Read the model definition and answer for the solid it produces. Units are mm, in the model's axes. Round coordinates to 2 decimals unless told otherwise and drop trailing zeros. Order: outer loops, then holes, each group sorted by start corner. A loop starts at its lowest first (then second) coordinate and runs counter-clockwise, first axis right, second up. Notation, with made-up numbers: (10.25, 70) -> (68.25, 70) arc R9 cw to (68.25, 75) -> close; hole circle Ø2 at (-1, 53). An arc over 180 degrees is marked (long way). Use a Markdown table: item, result. Add a question column.
1. Section C-C, the plane x = -8.5 is taken. Give the vertices of the cut face in (y, z).
2. Section D-D, the plane x = 59.5 is taken. Give the vertices of the cut face in (y, z).
3. Consider L1, parallel to Y at x = -7.5, z = 3.95; L2, parallel to Y at x = 8, z = 3.8; L3, parallel to Y at x = -13.5, z = 3.3. Determine where each line is inside the solid, lowest interval first. Write a range as [from, to].
4. Section A-A, the plane x = 12.5 is taken. Give the vertices of the cut face in (y, z).
5. Given pin 1 (2.5 mm diameter, centred on y = -155, z = 2, fed in from +X); pin 2 (2.5 mm diameter, centred on x = -36, z = 2.5, fed in from -Y); pin 3 (2 mm diameter, centred on x = -61.5, z = 3, fed in from -Y); pin 4 (2.5 mm diameter, centred on x = -63.46, y = -187.43, fed in from +Z), each flat-ended and moving along its own axis, determine where each tip first touches the part or whether it passes through.
6. Section B-B, the plane z = 2.8 is taken. Give the number of separate pieces and of enclosed holes in the cut face, then the cut area to 3 significant figures.
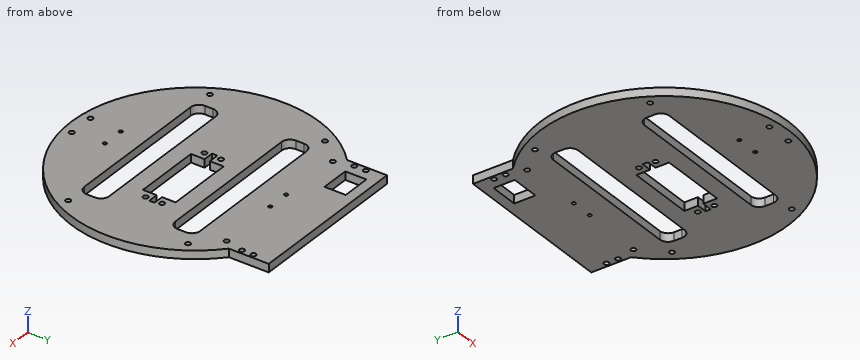
```python
from build123d import *

# Parameters (mm, degrees)
RESSALTO_EXTRUS_O1_DEPTH = 5
ESBO_O2_R                = 1.5
CORTE_EXTRUS_O1_DEPTH    = 10
ESBO_O3_W                = 6.3
ESBO_O3_H                = 3.2
ESBO_O3_R                = 1.5
CORTE_EXTRUS_O2_DEPTH    = 10
ESBO_O4_W                = 17.5
ESBO_O4_H                = 12.8
CORTE_EXTRUS_O3_DEPTH    = 6
ESBO_O5_R                = 1.5
CORTE_EXTRUS_O4_DEPTH    = 10
ESBO_O6_R                = 1.05
CORTE_EXTRUS_O5_DEPTH    = 10
CORTE_EXTRUS_O6_DEPTH    = 6


with BuildPart() as part:
    # Esboço1 → Ressalto-extrusão1 (new body)
    with BuildSketch(Plane.XY):
        with BuildLine():
            Line((44.495405461, -168.430491325), (44.495405461, -144.332190763))
            Line((44.495405461, -144.332190763), (-55.573351401, -144.332190763))
            Line((-55.573351401, -144.332190763), (-55.573351401, -168.393072388))
            Line((-55.573351401, -168.393072388), (-55.504594539, -168.430491325))
            ThreePointArc((-55.504594539, -168.430491325), (-5.504594539, -299.332190763), (44.495405461, -168.430491325))
        make_face()
    extrude(amount=RESSALTO_EXTRUS_O1_DEPTH)

    # Esboço2 → Corte-extrusão1 (cut)
    with BuildSketch(Plane.XY.offset(5)):
        with Locations((39.44625518, -173.430491325)):
            Circle(ESBO_O2_R)
        with Locations((52.44625518, -187.430491325)):
            Circle(ESBO_O2_R)
        with Locations((54.44625518, -258.430491325)):
            Circle(ESBO_O2_R)
        with Locations((-13.455444258, -293.430491325)):
            Circle(ESBO_O2_R)
        with Locations((2.44625518, -293.430491325)):
            Circle(ESBO_O2_R)
        with Locations((-65.455444258, -258.430491325)):
            Circle(ESBO_O2_R)
        with Locations((-63.455444258, -187.430491325)):
            Circle(ESBO_O2_R)
        with Locations((-50.455444258, -173.430491325)):
            Circle(ESBO_O2_R)
    extrude(amount=-CORTE_EXTRUS_O1_DEPTH, mode=Mode.SUBTRACT)

    # Esboço3 → Corte-extrusão2 (cut)
    with BuildSketch(Plane.XY.offset(5)):
        with Locations((28.245405461, -224.332190763)):
            Rectangle(ESBO_O3_W, ESBO_O3_H)
        Polygon((-21.804594539, -225.932190763), (-21.804594539, -222.732190763), (-15.504594539, -222.732190763), (-15.504594539, -214.432190763), (25.095405461, -214.432190763), (25.095405461, -234.232190763), (-15.504594539, -234.232190763), (-15.504594539, -225.932190763), align=None)
        with Locations((29.685405461, -229.332190763)):
            Circle(ESBO_O3_R)
        with Locations((29.685405461, -219.332190763)):
            Circle(ESBO_O3_R)
        with Locations((-20.094594539, -229.332190763)):
            Circle(ESBO_O3_R)
        with Locations((-20.094594539, -219.332190763)):
            Circle(ESBO_O3_R)
    extrude(amount=-CORTE_EXTRUS_O2_DEPTH, mode=Mode.SUBTRACT)

    # Esboço4 → Corte-extrusão3 (cut, through all)
    with BuildSketch(Plane.XY.offset(5)):
        with Locations((-37.823351401, -156.732190763)):
            Rectangle(ESBO_O4_W, ESBO_O4_H)
    extrude(amount=-CORTE_EXTRUS_O3_DEPTH, mode=Mode.SUBTRACT)

    # Esboço5 → Corte-extrusão4 (cut)
    with BuildSketch(Plane(origin=(0, 0, 0), x_dir=(-1, 0, 0), z_dir=(0, 0, -1))):
        with Locations((53.073351401, -155.332190763)):
            Circle(ESBO_O5_R)
        with Locations((53.073351401, -162.332190763)):
            Circle(ESBO_O5_R)
        with Locations((-41.995405461, -155.332190763)):
            Circle(ESBO_O5_R)
        with Locations((-41.995405461, -162.332190763)):
            Circle(ESBO_O5_R)
    extrude(amount=-CORTE_EXTRUS_O4_DEPTH, mode=Mode.SUBTRACT)

    # Esboço6 → Corte-extrusão5 (cut)
    with BuildSketch(Plane(origin=(0, 0, 0), x_dir=(-1, 0, 0), z_dir=(0, 0, -1))):
        with Locations((12.234594539, -174.332190763)):
            Circle(ESBO_O6_R)
        with Locations((-1.225405461, -174.332190763)):
            Circle(ESBO_O6_R)
        with Locations((-1.225405461, -274.332190763)):
            Circle(ESBO_O6_R)
        with Locations((12.234594539, -274.332190763)):
            Circle(ESBO_O6_R)
    extrude(amount=-CORTE_EXTRUS_O5_DEPTH, mode=Mode.SUBTRACT)

    # Esboço7 → Corte-extrusão6 (cut, through all)
    with BuildSketch(Plane(origin=(0, 0, 0), x_dir=(-1, 0, 0), z_dir=(0, 0, -1))):
        with BuildLine():
            Line((55.504594539, -254.332190763), (55.504594539, -249.332190763))
            ThreePointArc((55.504594539, -249.332190763), (54.040128445, -245.796656857), (50.504594539, -244.332190763))
            Line((50.504594539, -244.332190763), (-39.495405461, -244.332190763))
            ThreePointArc((-39.495405461, -244.332190763), (-43.030939367, -245.796656857), (-44.495405461, -249.332190763))
            Line((-44.495405461, -249.332190763), (-44.495405461, -254.332190763))
            ThreePointArc((-44.495405461, -254.332190763), (-43.030939367, -257.867724668), (-39.495405461, -259.332190763))
            Line((-39.495405461, -259.332190763), (50.504594539, -259.332190763))
            ThreePointArc((50.504594539, -259.332190763), (54.040128445, -257.867724668), (55.504594539, -254.332190763))
        make_face()
        with BuildLine():
            ThreePointArc((-39.495405461, -204.332190763), (-43.030939367, -202.867724668), (-44.495405461, -199.332190763))
            Line((-44.495405461, -199.332190763), (-44.495405461, -194.332190763))
            ThreePointArc((-44.495405461, -194.332190763), (-43.030939367, -190.796656857), (-39.495405461, -189.332190763))
            Line((-39.495405461, -189.332190763), (50.504594539, -189.332190763))
            ThreePointArc((50.504594539, -189.332190763), (54.040128445, -190.796656857), (55.504594539, -194.332190763))
            Line((55.504594539, -194.332190763), (55.504594539, -199.332190763))
            ThreePointArc((55.504594539, -199.332190763), (54.040128445, -202.867724668), (50.504594539, -204.332190763))
            Line((50.504594539, -204.332190763), (-39.495405461, -204.332190763))
        make_face()
    extrude(amount=-CORTE_EXTRUS_O6_DEPTH, mode=Mode.SUBTRACT)


solid = part.part
```
Verdict:
| question | item | result |
|---|---|---|
| 1 | outline | (-299.27, 0) -> (-259.33, 0) -> (-259.33, 5) -> (-299.27, 5) -> close; (-244.33, 0) -> (-234.23, 0) -> (-234.23, 5) -> (-244.33, 5) -> close; (-214.43, 0) -> (-204.33, 0) -> (-204.33, 5) -> (-214.43, 5) -> close; (-189.33, 0) -> (-144.33, 0) -> (-144.33, 5) -> (-189.33, 5) -> close |
| 2 | outline | (-261.74, 0) -> (-186.92, 0) -> (-186.92, 5) -> (-261.74, 5) -> close |
| 3 | L1 | y = [-299.31, -259.33], [-244.33, -234.23], [-214.43, -204.33], [-189.33, -144.33] |
| 3 | L2 | y = [-298.11, -259.33], [-244.33, -234.23], [-214.43, -204.33], [-189.33, -144.33] |
| 3 | L3 | y = [-298.9, -294.93], [-291.93, -259.33], [-244.33, -234.23], [-214.43, -204.33], [-189.33, -144.33] |
| 4 | outline | (-297.14, 0) -> (-259.33, 0) -> (-259.33, 5) -> (-297.14, 5) -> close; (-244.33, 0) -> (-234.23, 0) -> (-234.23, 5) -> (-244.33, 5) -> close; (-214.43, 0) -> (-204.33, 0) -> (-204.33, 5) -> (-214.43, 5) -> close; (-189.33, 0) -> (-144.33, 0) -> (-144.33, 5) -> (-189.33, 5) -> close |
| 5 | pin 1 | stops at x = 44.5 |
| 5 | pin 2 | stops at y = -293.4 |
| 5 | pin 3 | stops at y = -275.33 |
| 5 | pin 4 | passes through |
| 6 | separate pieces | 1 |
| 6 | enclosed holes | 24 |
| 6 | area | 14,600 mm2 |
